Here's the drawing with two shaded views (mm, measured from the low corner). I have some questions. A direction names the side the tool comes from. Give positions to 0.01 mm unless a question says otherwise; leave off trailing zeros. Write each loop counter-clockwise with the first axis right and the second up, starting at its lowest first coordinate (ties: lowest second). Pieces come first, ordered by that corner, then holes. Notation, with made-up numbers: (30.5, -5) -> (60.5, -5) arc R24 ccw to (60.5, 30) -> close; hole circle Ø9 at (31.5, 28). An arc over 180 degrees is marked (long way). One line per item, written item: value.
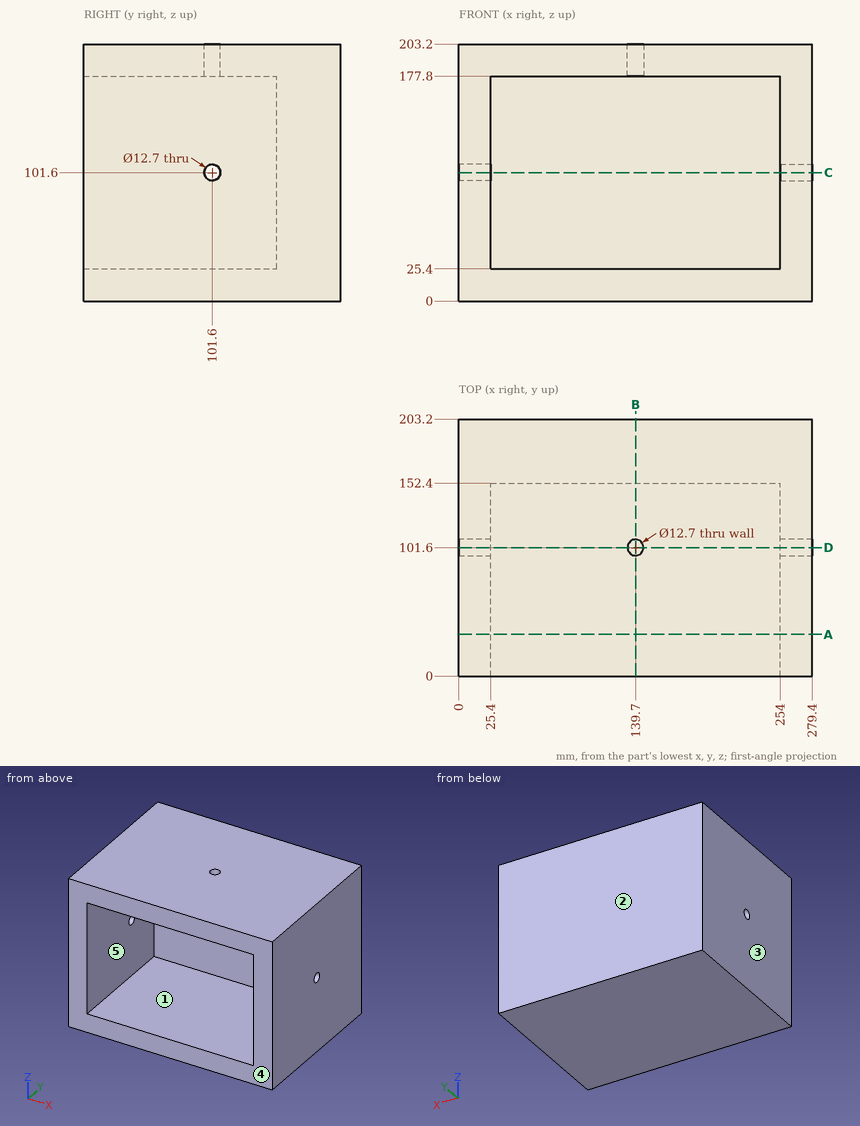
1) We'd pull the mould along X, two halves only. Please class the marked faces 1, 2 and 3: released by +X, released by -X, zero draft, split by the parting line, or undercut.
Answer list:
face 1: undercut
face 2: zero draft
face 3: released by -X
2) If we section it at A-A (y = 33): Write out the boundary of the cut face in (x, z).
Answer list:
outline: (0, 0) -> (279.4, 0) -> (279.4, 203.2) -> (0, 203.2) -> close; hole (25.4, 25.4) -> (254, 25.4) -> (254, 177.8) -> (25.4, 177.8) -> close
3) If we section it at D-D (y = 101.6): Write out the boundary of the cut face in (x, z).
Answer list:
outline: (0, 0) -> (279.4, 0) -> (279.4, 95.25) -> (254, 95.25) -> (254, 25.4) -> (25.4, 25.4) -> (25.4, 95.25) -> (0, 95.25) -> close; (0, 107.95) -> (25.4, 107.95) -> (25.4, 177.8) -> (133.35, 177.8) -> (133.35, 203.2) -> (0, 203.2) -> close; (146.05, 177.8) -> (254, 177.8) -> (254, 107.95) -> (279.4, 107.95) -> (279.4, 203.2) -> (146.05, 203.2) -> close
4) I need wall thicknesses on L1, parallel to Z at x = 234.5, y = 108; L2, parallel to X at y = 12.5, z = 149; L3, parallel to Z at x = 272, y = 101. Which ranges of each line are inside material? Lowest first, please.
Answer list:
L1: z = 0 to 25.4, 177.8 to 203.2
L2: x = 0 to 25.4, 254 to 279.4
L3: z = 0 to 95.28, 107.92 to 203.2
5) If we section it at C-C (z = 101.6): Write out the boundary of the cut face in (x, y), and give its area (3 significant figures).
Answer list:
outline: (0, 0) -> (25.4, 0) -> (25.4, 95.25) -> (0, 95.25) -> close; (0, 107.95) -> (25.4, 107.95) -> (25.4, 152.4) -> (254, 152.4) -> (254, 107.95) -> (279.4, 107.95) -> (279.4, 203.2) -> (0, 203.2) -> close; (254, 0) -> (279.4, 0) -> (279.4, 95.25) -> (254, 95.25) -> close
area: 21,300 mm^2
6) If we section it at B-B (x = 139.7): Write out the boundary of the cut face in (y, z), and give its area (3 significant figures).
Answer list:
outline: (0, 0) -> (203.2, 0) -> (203.2, 203.2) -> (107.95, 203.2) -> (107.95, 177.8) -> (152.4, 177.8) -> (152.4, 25.4) -> (0, 25.4) -> close; (0, 177.8) -> (95.25, 177.8) -> (95.25, 203.2) -> (0, 203.2) -> close
area: 17,700 mm^2
7) Will these pins go through, and if not, where does the flat tip stop? pin 1 (8 mm diameter, centred on x = 111.5, z = 68, fed in from -Y); pin 2 (11.5 mm diameter, centred on y = 101.6, z = 101.6, fed in from +X).
Answer list:
pin 1: stops at y = 152.4
pin 2: passes through
8) For the marked faces 4 and 5, which set-ups out of +Z, -Z, +X, -X, +Y, -Y let a thin tool reach every point of the face, with its end or its side?
Answer list:
face 4: +Z, -Z, +X, -X, -Y
face 5: -Y
